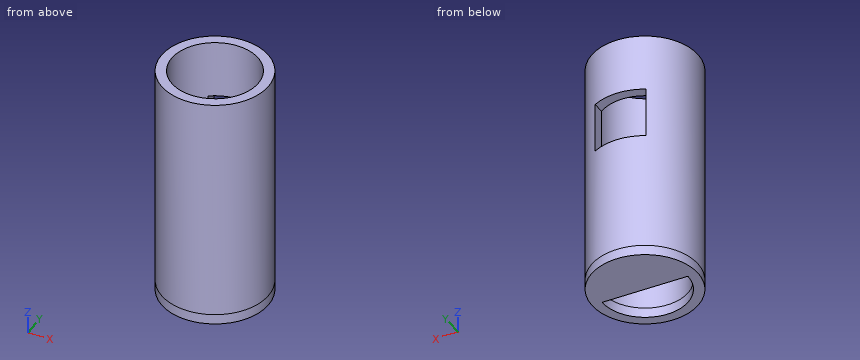
from build123d import *

# Parameters (mm, degrees)
SKETCH1_R           = 10.5
SKETCH1_R_2         = 8.5
BOSS_EXTRUDE1_DEPTH = 45
SKETCH2_W           = 10
SKETCH2_H           = 10
CUT_EXTRUDE1_DEPTH  = 40
BOSS_EXTRUDE4_START = 2
SKETCH6_R           = 10.5
BOSS_EXTRUDE4_DEPTH = 2


with BuildPart() as part:
    # Sketch1 → Boss-Extrude1 (new body)
    with BuildSketch(Plane.XY):
        with Locations(Location((0, 0, 0), (0, 0, 180))):
            Circle(SKETCH1_R)
        with Locations(Location((0, 0, 0), (0, 0, 180))):
            Circle(SKETCH1_R_2, mode=Mode.SUBTRACT)
    extrude(amount=BOSS_EXTRUDE1_DEPTH)

    # Sketch2 → Cut-Extrude1 (cut)
    with BuildSketch(Plane(origin=(0, 0, 0), x_dir=(1, 0, 0), z_dir=(0, 1, 0))):
        with Locations((0, -28.58915915)):
            Rectangle(SKETCH2_W, SKETCH2_H)
    extrude(amount=CUT_EXTRUDE1_DEPTH, mode=Mode.SUBTRACT)

    # Sketch6 → Boss-Extrude4 (add)
    with BuildSketch(Plane(origin=(0, 0, 0), x_dir=(-1, 0, 0), z_dir=(0, 0, -1)).offset(BOSS_EXTRUDE4_START)):
        Circle(SKETCH6_R)
        with BuildLine():
            Line((-8.5, 0), (8.5, 0))
            ThreePointArc((8.5, 0), (0, -8.5), (-8.5, 0))
        make_face(mode=Mode.SUBTRACT)
    extrude(amount=-BOSS_EXTRUDE4_DEPTH)


solid = part.part
Verification items for the finished model (mm, model axes). Give positions to 0.01 mm unless a question says otherwise; leave off trailing zeros. Write each loop counter-clockwise with the first axis right and the second up, starting at its lowest first coordinate (ties: lowest second). Pieces come first, ordered by that corner, then holes.
(1) Cross-section at C-C (x = 7). Enter the section's corners in (y, z).
(2) Cross-section at B-B (y = -4). Enter the section's corners in (x, z), plus the area to 3 significant figures.
(3) Material ranges on line 1 (Y direction, x = 0, z = 21); line 2 (Z direction, x = -4.5, y = 4.5); line 3 (X direction, y = 1, z = 23), recorded low to high.
(4) Cross-section at D-D (z = 18.5). Enter the section's corners in (x, y).
(5) Cross-section at A-A (x = 0). Enter the section's corners in (y, z), plus the area to 3 significant figures.
(6) Gauge pin test, flat ends, axial feed: pin 1 (1 mm diameter, centred on y = 3.5, z = 28.5, fed in from +X); pin 2 (1.2 mm diameter, centred on y = 7.5, z = 30, fed in from -X); pin 3 (1.9 mm diameter, centred on y = 8.5, z = 28, fed in from +X). Record the tip position at first contact, or that the pin passes through.
Worked out:
1. outline: (-7.83, -2) - (-4.82, -2) - (-4.82, 45) - (-7.83, 45) - close; (0, -2) - (7.83, -2) - (7.83, 45) - (4.82, 45) - (4.82, 0) - (0, 0) - close
2. outline: (-9.71, -2) - (-7.5, -2) - (-7.5, 45) - (-9.71, 45) - close; (7.5, -2) - (9.71, -2) - (9.71, 45) - (7.5, 45) - close
2. area: 208 mm2
3. line 1: y = -10.5 to -8.5, 8.5 to 10.5
3. line 2: z = -2 to 0
3. line 3: x = -10.45 to -8.44, 8.44 to 10.45
4. outline: circle Ø21 at (0, 0); hole circle Ø17 at (0, 0)
5. outline: (-10.5, -2) - (-8.5, -2) - (-8.5, 45) - (-10.5, 45) - close; (0, -2) - (10.5, -2) - (10.5, 23.59) - (8.5, 23.59) - (8.5, 0) - (0, 0) - close; (8.5, 33.59) - (10.5, 33.59) - (10.5, 45) - (8.5, 45) - close
5. area: 185 mm2
6. pin 1: stops at x = 10.06
6. pin 2: stops at x = -7.91
6. pin 3: stops at x = 7.3
